The listing builds one solid part. Answer for the finished solid, in the listing's coordinates (mm). Coordinates: 2 decimals unless noted, no trailing zeros. Order: outer loops, then holes, each group sorted by start corner. A loop starts at its lowest first (then second) coordinate and runs counter-clockwise, first axis right, second up. Notation, with made-up numbers: (70.5, 36.25) -> (102.5, 36.25) arc R19 cw to (102.5, 49.25) -> close; hole circle Ø3 at (8.5, 7.5). An arc over 180 degrees is marked (long way). One line per question, with ' | ' between items.
Autodesk Inventor part; units mm, degrees
ref_plane "YZ Plane" through (0, 0, 0) normal (1, 0, 0) x (0, 1, 0)
ref_plane "XZ Plane" through (0, 0, 0) normal (0, 1, 0) x (-1, 0, 0)
ref_plane "XY Plane" through (0, 0, 0) normal (0, 0, 1) x (1, 0, 0)
sketch "Sketch1" plane through (0, 0, 0) normal (0, 0, 1) x (1, 0, 0)
  line L0 (0, 0) -> (0, -23.75)
  line L1 (0, -23.75) -> (6, -23.75)
  line L2 (6, 0) -> (6, -23.75)
  line L3 (0, 0) -> (6, 0)
  line L4 (0, -23.75) -> (0, -58.75)
  line L5 (0, -58.75) -> (6, -58.75)
  line L6 (6, -23.75) -> (6, -58.75) construction
  line L7 (0, -23.75) -> (6, -23.75)
  line L8 (0, -58.75) -> (0, -82.5)
  line L9 (0, -82.5) -> (6, -82.5)
  line L10 (6, -58.75) -> (6, -82.5)
  line L11 (0, -58.75) -> (6, -58.75)
  line L12 (0, -82.5) -> (0, -117.5)
  line L13 (0, -117.5) -> (6, -117.5)
  line L14 (6, -82.5) -> (6, -117.5) construction
  line L15 (0, -82.5) -> (6, -82.5)
  line L16 (0, -117.5) -> (0, -136.6283)
  line L17 (0, -136.6283) -> (6, -136.6283)
  line L18 (6, -117.5) -> (6, -136.6283)
  line L19 (0, -117.5) -> (6, -117.5)
  line L20 (0, -136.6283) -> (0, -171.6283)
  line L21 (0, -171.6283) -> (6, -171.6283)
  line L22 (6, -136.6283) -> (6, -171.6283) construction
  line L23 (0, -136.6283) -> (6, -136.6283)
  line L24 (0, -171.6283) -> (0, -200)
  line L25 (0, -200) -> (6, -200)
  line L26 (6, -171.6283) -> (6, -200)
  line L27 (0, -171.6283) -> (6, -171.6283)
  line L28 (0, -200) -> (40, -200)
  line L29 (40, -200) -> (40, 0)
  line L30 (40, 0) -> (0, 0)
  line L31 (0, 0) -> (0, -200)
extrude "Extrusion1" add sketch "Sketch1" against normal blind 6 contours L1 L2 L30 L29 L28 L26 L21 L20 L17 L18 L13 L12 L9 L10 L5 L4
sketch "Sketch2" plane through (0, 0, 0) normal (0, 0, 1) x (1, 0, 0)
  line L0 (6, 0) -> (6, -23.75) construction
  line L1 (6, -23.75) -> (0, -23.75) construction
  line L2 (0, -23.75) -> (0, -58.75) construction
  line L3 (0, -58.75) -> (6, -58.75) construction
  line L4 (6, -58.75) -> (6, -82.5) construction
  line L5 (0, -82.5) -> (6, -82.5) construction
  line L6 (0, -82.5) -> (0, -117.5) construction
  line L7 (0, -117.5) -> (6, -117.5) construction
  line L8 (6, -117.5) -> (6, -136.6283) construction
  line L9 (0, -136.6283) -> (6, -136.6283) construction
  line L10 (0, -136.6283) -> (0, -171.6283) construction
  line L11 (0, -171.6283) -> (6, -171.6283) construction
  line L12 (6, -171.6283) -> (6, -200) construction
  line L13 (40, 0) -> (40, -200) construction
  line L14 (40, -156.4035) -> (0, -156.4035) construction
  line L15 (0, -171.6283) -> (0, -136.6283) construction
  line L16 (20, -156.4035) -> (20, -119.6077) construction
  line L17 (34, 0) -> (34, -23.75)
  line L18 (34, -23.75) -> (40, -23.75)
  line L19 (40, -23.75) -> (40, -58.75)
  line L20 (40, -58.75) -> (34, -58.75)
  line L21 (34, -58.75) -> (34, -82.5)
  line L22 (40, -82.5) -> (34, -82.5)
  line L23 (40, -82.5) -> (40, -117.5)
  line L24 (40, -117.5) -> (34, -117.5)
  line L25 (34, -117.5) -> (34, -136.6283)
  line L26 (40, -136.6283) -> (34, -136.6283)
  line L27 (40, -136.6283) -> (40, -171.6283) construction
  line L28 (40, -171.6283) -> (34, -171.6283)
  line L29 (34, -171.6283) -> (34, -200)
  line L30 (0, -156.4035) -> (40, -156.4035) construction
  line L31 (40, -171.6283) -> (40, -136.6283) construction
  line L32 (40, 0) -> (40, -200) construction
  line L33 (40, -200) -> (6, -200) construction
  line L34 (34, -200) -> (40, -200)
  line L35 (6, 0) -> (40, 0) construction
  line L36 (34, 0) -> (40, 0)
  line L37 (40, -117.5) -> (40, -136.6283)
  line L38 (40, -171.6283) -> (40, -200)
  line L39 (40, 0) -> (40, -23.75)
  line L40 (40, -82.5) -> (40, -58.75)
  point P0 (0, 0)
extrude "Extrusion2" cut sketch "Sketch2" against normal through all
properties part number "front"
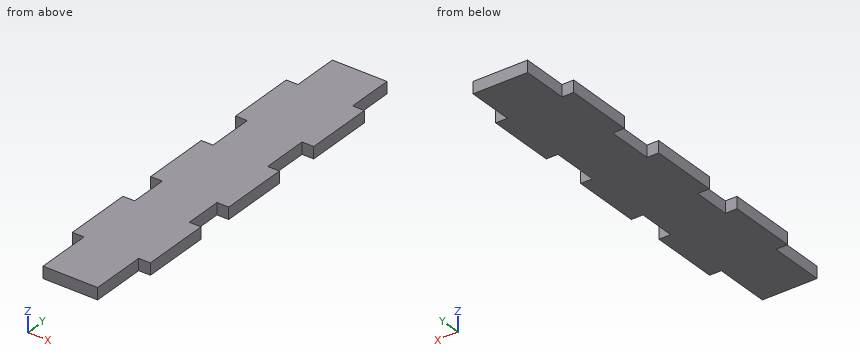
Item 1: Section A-A, the plane z = -2.45 is taken. Give the vertices of the cut face in (x, y).
Computed values:
outline: (0, -171.63) -> (6, -171.63) -> (6, -200) -> (34, -200) -> (34, -171.63) -> (40, -171.63) -> (40, -136.63) -> (34, -136.63) -> (34, -117.5) -> (40, -117.5) -> (40, -82.5) -> (34, -82.5) -> (34, -58.75) -> (40, -58.75) -> (40, -23.75) -> (34, -23.75) -> (34, 0) -> (6, 0) -> (6, -23.75) -> (0, -23.75) -> (0, -58.75) -> (6, -58.75) -> (6, -82.5) -> (0, -82.5) -> (0, -117.5) -> (6, -117.5) -> (6, -136.63) -> (0, -136.63) -> close
Item 2: Each of these flat-tipped pins is pushed along its axis until it touches: pin 1 Ø1.8 at (x, z) = (36.5, -4.5) entering from -Y; pin 2 Ø1.8 at (y, z) = (-126, -2) entering from -X; pin 3 Ø2 at (x, y) = (33, -80.5) entering from +Z; pin 4 Ø3 at (y, z) = (-69, -3.5) entering from +X. Where does it stop, or does it pass through?
Computed values:
pin 1: stops at y = -171.63 | pin 2: stops at x = 6 | pin 3: stops at z = 0 | pin 4: stops at x = 34
Item 3: Section B-B, the plane y = -133 is taken. Give the vertices of the cut face in (x, z), plus the area to 3 significant figures.
Computed values:
outline: (6, -6) -> (34, -6) -> (34, 0) -> (6, 0) -> close | area: 168 mm^2
Item 4: Find the intervals of material crossed by L1, parallel to Y at x = 3, z = -3.6; L2, parallel to X at y = -173, z = -4.7, in increasing order.
Computed values:
L1: y = -171.63 to -136.63, -117.5 to -82.5, -58.75 to -23.75 | L2: x = 6 to 34
